```python
from build123d import *

# Parameters (mm, degrees)
F0_W      = 1117.6
F0_H      = 406.4
F1_DEPTH  = 19.05
F2_W      = 63.5
F2_H      = 63.5
F3_DEPTH  = 457.2
F6_W      = 19.05
F6_H      = 228.6
F7_DEPTH  = 82.55
F9_W      = 914.4
F9_H      = 19.05
F10_DEPTH = 82.55
F11_W     = 914.4
F11_H     = 15.875
F12_DEPTH = 82.55
F13_W     = 292.1707866669
F13_H     = 82.55
F14_DEPTH = 19.05
F15_W     = 292.3078624487
F15_H     = 82.55
F16_DEPTH = 19.05
F17_W     = 19.05
F17_H     = 292.1
F18_DEPTH = 82.55
F19_W     = 19.05
F19_H     = 292.1
F20_DEPTH = 82.55
F21_W     = 19.05
F21_H     = 292.1
F22_DEPTH = 82.55


with BuildPart() as f1:
    # F0 (on Top) → F1 (new body)
    with BuildSketch(Plane.XY):
        Rectangle(F0_W, F0_H)
    extrude(amount=F1_DEPTH)

    # F2 (on face) → F3 (join)
    with BuildSketch(Plane(origin=(0, 0, 0), x_dir=(1, 0, 0), z_dir=(0, 0, -1))):
        with Locations((-488.95, 146.05)):
            Rectangle(F2_W, F2_H)
    extrude(amount=F3_DEPTH)

    # F4: F1 across plane


with BuildPart() as f1_1:
    add(f1.part)
    add(f1.part.mirror(Plane.XZ))

    # F5: F1 across plane


with BuildPart() as f1_2:
    add(f1_1.part)
    add(f1_1.part.mirror(Plane.YZ))

    # F6 (on face) → F7 (join)
    with BuildSketch(Plane(origin=(0, 0, 0), x_dir=(1, 0, 0), z_dir=(0, 0, -1))):
        with Locations((495.3, 0)):
            Rectangle(F6_W, F6_H)
    extrude(amount=F7_DEPTH)

    # F8: F1 across plane


with BuildPart() as f1_3:
    add(f1_2.part)
    add(f1_2.part.mirror(Plane.YZ))

    # F9 (on face) → F10 (join)
    with BuildSketch(Plane(origin=(0, 0, 0), x_dir=(1, 0, 0), z_dir=(0, 0, -1))):
        with Locations((0, -155.575)):
            Rectangle(F9_W, F9_H)
    extrude(amount=F10_DEPTH)

    # F11 (on face) → F12 (join)
    with BuildSketch(Plane(origin=(0, 0, 0), x_dir=(1, 0, 0), z_dir=(0, 0, -1))):
        with Locations((0, 153.9875)):
            Rectangle(F11_W, F11_H)
    extrude(amount=F12_DEPTH)

    # F13 (on face) → F14 (join)
    with BuildSketch(Plane(origin=(457.2, 0, 0), x_dir=(0, -1, 0), z_dir=(-1, 0, 0))):
        with Locations((0.0353933334, -41.275)):
            Rectangle(F13_W, F13_H)
    extrude(amount=F14_DEPTH)

    # F15 (on face) → F16 (join)
    with BuildSketch(Plane.YZ.offset(-457.2)):
        with Locations((0.1039312243, -41.275)):
            Rectangle(F15_W, F15_H)
    extrude(amount=F16_DEPTH)

    # F17 (on face) → F18 (join)
    with BuildSketch(Plane(origin=(0, 0, 0), x_dir=(1, 0, 0), z_dir=(0, 0, -1))):
        Rectangle(F17_W, F17_H)
    extrude(amount=F18_DEPTH)

    # F19 (on face) → F20 (join)
    with BuildSketch(Plane(origin=(0, 0, 0), x_dir=(1, 0, 0), z_dir=(0, 0, -1))):
        with Locations((-233.3625, 0)):
            Rectangle(F19_W, F19_H)
    extrude(amount=F20_DEPTH)

    # F21 (on face) → F22 (join)
    with BuildSketch(Plane(origin=(0, 0, 0), x_dir=(1, 0, 0), z_dir=(0, 0, -1))):
        with Locations((223.8375, 0)):
            Rectangle(F21_W, F21_H)
    extrude(amount=F22_DEPTH)


solid = f1_3.part
```
Geometry: final body of the model. Coordinates: model frame, mm. A direction names the side the tool comes from. Give positions to 0.01 mm unless a question says otherwise; leave off trailing zeros. Order: outer loops, then holes, each group sorted by start corner. A loop starts at its lowest first (then second) coordinate and runs counter-clockwise, first axis right, second up. Notation, with made-up numbers: M -6,-12.5 L 16,-12.5 A23 ccw 16,23.5 Z; hole C 18,-13.5 d10. An arc over 180 degrees is marked long. Answer as CSV lines item,"result". Start each with the question number.
1) First-contact query: P1, Ø10, axis at x = 231, y = -58, coming from the -Z side; P2, Ø19, axis at y = 138, z = -211, coming from the +X side; P3, Ø6, axis at x = -361.5, y = -107, coming from the -Z side. Flat tips, straight axial feed; report the tip coordinate or a pass-through.
2) Mould query, pull axis X, two halves, no side actions, for faces 4 (the flat face through (-472, 2, 0)), 5 (the flat face through (520.7, 146, -225)), 6 (the flat face through (489, 146, -457.2)). Classes: +X half, -X half, draft (parallel to the pull), parting line (faces both ways), or undercut.
3) Cut plane A-A (x = 368). Output: boundary loops of the cut face in (y, z) (3 decimals), then the cut area to 3 significant figures.
4) Cut plane B-B (z = -121.5). Output: boundary loops of the cut face in (x, y), then the cut area to 3 significant figures.
5) Line query: line 1 (Y direction, x = -173, z = -26) (3 decimals); line 2 (Z direction, x = -391, y = -3). Output: solid intervals per line, ascending. Write a range as from..to.
6) Cut plane D-D (z = -58). State how many separate pieces and enclosed holes the cut face has, then the cut area to 3 significant figures.
7) Set-up query: faces 1 (the flat face through (-242.888, 2, -41)), 2 (the flat face through (489, -177.8, -225)), 3 (the flat face through (489, 177.8, -225)). Return all of +Z, -Z, +X, -X, +Y, -Y with unobstructed straight access to the full face (end or side cutting, diameter ignored); none if empty.
Findings below:
1,P1,"stops at z = -82.55"
1,P2,"stops at x = 520.7"
1,P3,"stops at z = 0"
2,face 4,"undercut"
2,face 5,"+X half"
2,face 6,"draft"
3,outline,"M -203.2,0 L -161.925,0 L -161.925,-82.55 L -146.05,-82.55 L -146.05,0 L 146.05,0 L 146.05,-82.55 L 165.1,-82.55 L 165.1,0 L 203.2,0 L 203.2,19.05 L -203.2,19.05 Z"
3,area,"10,600 mm²"
4,outline,"M -520.7,-177.8 L -457.2,-177.8 L -457.2,-114.3 L -520.7,-114.3 Z; M -520.7,114.3 L -457.2,114.3 L -457.2,177.8 L -520.7,177.8 Z; M 457.2,-177.8 L 520.7,-177.8 L 520.7,-114.3 L 457.2,-114.3 Z; M 457.2,114.3 L 520.7,114.3 L 520.7,177.8 L 457.2,177.8 Z"
4,area,"16,100 mm²"
5,line 1,"y = -161.925..-146.05, 146.05..165.1"
5,line 2,"z = 0..19.05"
6,separate pieces,"1"
6,enclosed holes,"6"
6,area,"84,600 mm²"
7,face 1,"-Z"
7,face 2,"-Z, +X, -X, -Y"
7,face 3,"-Z, +X, -X, +Y"
